Input: part model. Units: mm. Frame: model coordinates. A direction names the side the tool comes from. Coordinates: 2 decimals unless noted, no trailing zeros. Order: outer loops, then holes, each group sorted by start corner. A loop starts at its lowest first (then second) coordinate and runs counter-clockwise, first axis right, second up. Notation, with made-up numbers: M -7.75,-38 L 39.25,-38 A24 cw 39.25,-19 Z; hole C 17,38 d6. An arc over 180 degrees is marked long. Answer in a Markdown table with one row per item.
from build123d import *

# Parameters (mm, degrees)
F0_W     = 7.9375
F0_H     = 33.3375
F0_R     = 1.35255
F1_DEPTH = 11.9827929
F2_R     = 3.96874
F3_R     = 4.7625
F4_R     = 1.7272
F5_DEPTH = 7.9375
F6_R     = 3.175
F6_R_2   = 1.7272
F8_DEPTH = 4.7625


# Not quite as in the source:
# - a fillet or chamfer is up to 0.001 mm smaller than in the source, because OpenCascade refuses the exact size


with BuildPart() as f1:
    # F0 (on Top) → F1 (new body)
    with BuildSketch(Plane.XY):
        with Locations((3.96875, 16.66875)):
            Rectangle(F0_W, F0_H)
        with Locations((3.96875, 13.49375)):
            Circle(F0_R, mode=Mode.SUBTRACT)
        with Locations((3.96875, 29.36875)):
            Circle(F0_R, mode=Mode.SUBTRACT)
    extrude(amount=F1_DEPTH)

    # F2 (radius 3.96875 in the source; OpenCascade refuses exactly that, so slightly less here)
    f2_edges = [f1.edges().sort_by_distance(p)[0] for p in [
        (7.9375, 33.3375, 5.991396),
        (0, 33.3375, 5.991396),
    ]]
    fillet(f2_edges, radius=F2_R)

    # F3
    f3_edges = [f1.edges().sort_by_distance(p)[0] for p in [
        (3.96875, 0, 11.982793),
    ]]
    fillet(f3_edges, radius=F3_R)

    # F4 (on face) → F5 (cut, through all)
    with BuildSketch(Plane.YZ.offset(7.9375)):
        with Locations((4.7625, 7.2202929)):
            Circle(F4_R)
    extrude(amount=-F5_DEPTH, mode=Mode.SUBTRACT)

    # F6 (on face) → F8 (cut, through all)
    with BuildSketch(Plane(origin=(0, 0, 0), x_dir=(0, -1, 0), z_dir=(-1, 0, 0))):
        with Locations((-4.7625, 7.2202929)):
            Circle(F6_R)
        with Locations((-4.7625, 7.2202929)):
            Circle(F6_R_2, mode=Mode.SUBTRACT)
    extrude(amount=-F8_DEPTH, mode=Mode.SUBTRACT)


solid = f1.part
1) Material intervals for probe 1 along Y at (x, z) = (3.5, 9); probe 2 along X at (y, z) = (13.5, 10.5); probe 3 along Y at (x, z) = (4.25, 2.5), sorted ascending.
Resolved:
| item | result |
|---|---|
| probe 1 | y = 0.35 to 2.13, 7.39 to 12.23, 14.76 to 28.1, 30.64 to 33.31 |
| probe 2 | x = 0 to 2.62, 5.32 to 7.94 |
| probe 3 | y = 0 to 12.17, 14.82 to 28.05, 30.69 to 33.33 |
2) Contact query for flat-ended pins moving along their axis: pin 1 (5 mm diameter, centred on y = 4.5, z = 9, fed in from -X); pin 2 (4 mm diameter, centred on x = 6.5, z = 10.5, fed in from -Y); pin 3 (4.5 mm diameter, centred on y = 4.76, z = 7.22, fed in from -X); pin 4 (2 mm diameter, centred on x = 3.97, y = 13.49, fed in from +Z). Output: stop coordinate, or through.
Resolved:
| item | result |
|---|---|
| pin 1 | stops at x = 0 |
| pin 2 | stops at y = 0.18 |
| pin 3 | stops at x = 4.76 |
| pin 4 | passes through |
3) Reachability of faces 1 (the face through (4.762, 3, 6)), 2 (the face through (3.793, 14.835, 5.908)) from +Z, -Z, +X, -X, +Y, -Y: full face, straight path, thin tool, end or side. Return the list, or none.
Resolved:
| item | result |
|---|---|
| face 1 | -X |
| face 2 | +Z, -Z |
4) Cut plane C-C, the plane y = 12.5. Output: boundary loops of the cut face in (x, z), and give its area (3 significant figures).
Resolved:
| item | result |
|---|---|
| outline | M 0,0 L 3.05,0 L 3.05,11.98 L 0,11.98 Z; M 4.89,0 L 7.94,0 L 7.94,11.98 L 4.89,11.98 Z |
| area | 73.1 mm2 |
5) Mould query, pull axis Z, two halves, no side actions, for faces 3 (the face through (2.348, 1.734, 8.174)), 4 (the face through (4, 0, 4)), 5 (the face through (4, 17, 0)). Classes: +Z half, -Z half, draft (parallel to the pull), parting line (faces both ways), or undercut.
Resolved:
| item | result |
|---|---|
| face 3 | undercut |
| face 4 | draft |
| face 5 | -Z half |
6) Cut plane A-A, the plane z = 8. State how many separate pieces and enclosed holes the cut face has, and give its area (3 significant figures).
Resolved:
| item | result |
|---|---|
| separate pieces | 2 |
| enclosed holes | 2 |
| area | 207 mm2 |
